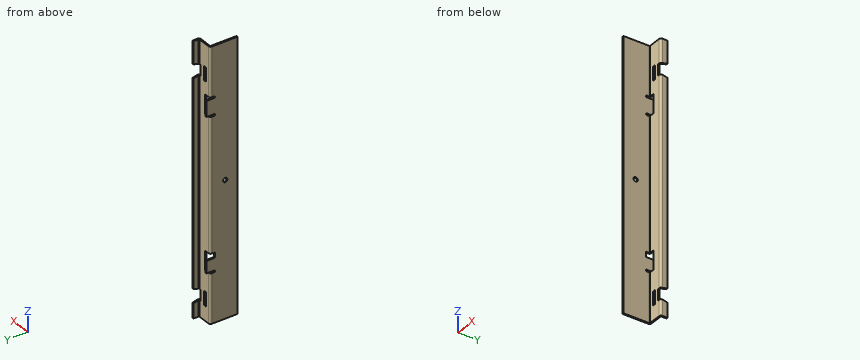
```python
from build123d import *

# Parameters (mm, degrees)
EXTRUDE1_DEPTH     = 247.65
FILLET2_R          = 1.27
FILLET3_R          = 3.81
SKETCH2_W          = 34.925
SKETCH2_H          = 9.525
CUT_EXTRUDE1_DEPTH = 12.7
SKETCH3_W          = 2.54
SKETCH3_H          = 22.225
SKETCH3_H_2        = 28.575
EXTRUDE2_DEPTH     = 15.875
FILLET1_R          = 1.5875
SKETCH4_W          = 4.953
SKETCH4_H          = 25.4
CUT_EXTRUDE2_DEPTH = 2.54
CUT_EXTRUDE3_DEPTH = 6.35
SKETCH6_R          = 3.96875
CUT_EXTRUDE4_DEPTH = 2.54


with BuildPart() as part:
    # Sketch1 → Extrude1 (new, symmetric)
    with BuildSketch(Plane.XY):
        Polygon((-3.512251891, 50.775495097), (-3.512251891, -0.183254903), (-0.972251891, -0.183254903), (-0.972251891, 48.235495097), (26.967748109, 48.235495097), (26.967748109, 61.094245097), (24.427748109, 61.094245097), (24.427748109, 50.775495097), align=None)
    extrude(amount=EXTRUDE1_DEPTH, both=True)

    # Fillet2
    fillet2_edges = [part.edges().sort_by_distance(p)[0] for p in [
        (24.427748109, 50.775495097, 0),
        (-0.972251891, 48.235495097, 0),
    ]]
    fillet(fillet2_edges, radius=FILLET2_R)

    # Fillet3
    fillet3_edges = [part.edges().sort_by_distance(p)[0] for p in [
        (26.967748109, 48.235495097, 0),
        (-3.512251891, 50.775495097, 0),
    ]]
    fillet(fillet3_edges, radius=FILLET3_R)

    # Sketch2 → Cut-Extrude1 (cut)
    with BuildSketch(Plane.ZY.offset(3.512251891)):
        with Locations((-139.7, 46.012995097)):
            Rectangle(SKETCH2_W, SKETCH2_H)
        with Locations((139.7, 46.012995097)):
            Rectangle(SKETCH2_W, SKETCH2_H)
    extrude(amount=-CUT_EXTRUDE1_DEPTH, mode=Mode.SUBTRACT)

    # Sketch3 → Extrude2 (add)
    with BuildSketch(Plane(origin=(0, 41.250495097, 0), x_dir=(1, 0, 0), z_dir=(0, 1, 0))):
        with Locations((-2.242251891, 142.875)):
            Rectangle(SKETCH3_W, SKETCH3_H)
        with Locations((-2.242251891, -139.7)):
            Rectangle(SKETCH3_W, SKETCH3_H_2)
    extrude(amount=EXTRUDE2_DEPTH)

    # Fillet1
    fillet1_edges = [part.edges().sort_by_distance(p)[0] for p in [
        (-2.242251891, 41.250495097, -153.9875),
        (-2.242251891, 41.250495097, -131.7625),
        (-2.242251891, 41.250495097, 125.4125),
        (-2.242251891, 41.250495097, 153.9875),
        (-2.242251891, 41.250495097, -157.1625),
        (-2.242251891, 41.250495097, 157.1625),
        (-2.242251891, 41.250495097, 122.2375),
    ]]
    fillet(fillet1_edges, radius=FILLET1_R - 0.0001)  # a hair under: the kernel refuses the full size

    # Sketch4 → Cut-Extrude2 (cut)
    with BuildSketch(Plane(origin=(0, 50.775495097, 0), x_dir=(1, 0, 0), z_dir=(0, 1, 0))):
        with Locations((9.632248109, 207.9625)):
            Rectangle(SKETCH4_W, SKETCH4_H)
        with Locations((9.632248109, -193.675)):
            Rectangle(SKETCH4_W, SKETCH4_H)
    extrude(amount=-CUT_EXTRUDE2_DEPTH, mode=Mode.SUBTRACT)

    # Sketch5 → Cut-Extrude3 (cut)
    with BuildSketch(Plane(origin=(26.967748109, 0, 0), x_dir=(0, 0, -1), z_dir=(1, 0, 0))):
        Polygon((195.2625, 61.094245097), (220.6625, 61.094245097), (218.28125, 52.045495097), (218.28125, 48.235495097), (197.64375, 48.235495097), (197.64375, 52.045495097), align=None)
        Polygon((-180.975, 61.094245097), (-206.375, 61.094245097), (-203.99375, 52.045495097), (-203.99375, 48.235495097), (-183.35625, 48.235495097), (-183.35625, 52.045495097), align=None)
    extrude(amount=-CUT_EXTRUDE3_DEPTH, mode=Mode.SUBTRACT)

    # Sketch6 → Cut-Extrude4 (cut)
    with BuildSketch(Plane.ZY.offset(3.512251891)):
        with Locations((0, 22.225)):
            Circle(SKETCH6_R)
    extrude(amount=-CUT_EXTRUDE4_DEPTH, mode=Mode.SUBTRACT)


solid = part.part
```
The model under review builds one solid part; all positions refer to its coordinate system, in mm. Coordinates: 2 decimals unless noted, no trailing zeros. Loops run counter-clockwise (first coordinate to the right, second up) from the corner with the lowest first, then second, coordinate; pieces in that order, holes last. Notation, with made-up numbers: (-25.75, -21.75) -> (29.25, -21.75) arc R23 cw to (29.25, -9.75) -> close; hole circle Ø4 at (82.5, -1). An arc over 180 degrees is marked (long way). Answer as CSV lines item,"result".
Item 1: Take a section at A-A, the plane z = 140. State the section outline as (x, y) points, and give its area (3 significant figures).
Results below:
outline,"(-3.51, -0.18) -> (-0.97, -0.18) -> (-0.97, 57.13) -> (-3.51, 57.13) -> close; (9.19, 48.24) -> (23.16, 48.24) arc R3.81 ccw to (26.97, 52.05) -> (26.97, 61.09) -> (24.43, 61.09) -> (24.43, 52.05) arc R1.27 cw to (23.16, 50.78) -> (9.19, 50.78) -> close"
area,"214 mm2"
Item 2: Insertion check: pin 1 (3 mm diameter, centred on x = -2.5, z = 135, fed in from +Y); pin 2 (0.8 mm diameter, centred on x = -2, y = 52, fed in from +Z); pin 3 (6 mm diameter, centred on x = 12, z = -117, fed in from -Y). Each pin has a flat end and moves straight along its axis. Give the tip position at first contact, or say it passes through.
Results below:
pin 1,"stops at y = 57.13"
pin 2,"stops at z = 153.99"
pin 3,"stops at y = 48.24"
Item 3: For L1, parallel to Y at x = 7.5, z = -21.5; L2, parallel to X at y = 43.5, z = 163.5; L3, parallel to Y at x = -2.2, z = 0, list the stretches that pass through material, from the lowest coordinate up.
Results below:
L1,"y = 48.24 to 50.78"
L2,"x = -3.51 to -0.97"
L3,"y = -0.18 to 18.26, 26.19 to 49.84"
Item 4: Take a section at B-B, the plane y = 12.5. State the section outline as (x, z) points, and give its area (3 significant figures).
Results below:
outline,"(-3.51, -247.65) -> (-0.97, -247.65) -> (-0.97, 247.65) -> (-3.51, 247.65) -> close"
area,"1,260 mm2"
